from build123d import *

# Parameters (mm, degrees)
FILLET1_R          = 0.508
CHAMFER1_SIZE      = 0.508
CHAMFER1_SIZE2     = 0.87988181
SKETCH4_W          = 19.05
SKETCH4_H          = 3.175
CUT_EXTRUDE1_DEPTH = 4.7625
FILLET2_R          = 1.5875


with BuildPart() as part:
    # Sketch3 → Revolve1 (revolve)
    with BuildSketch(Plane(origin=(0, 0, 0), x_dir=(0, 0, -1), z_dir=(1, 0, 0)), mode=Mode.PRIVATE) as revolve1_sk:
        with BuildLine():
            Line((0, 0), (3.175, 0))
            Line((3.175, 0), (3.175, -8.255))
            ThreePointArc((3.175, -8.255), (3.691804849, -12.180522558), (5.207, -15.838527241))
            Line((5.207, -15.838527241), (10.16, -24.417374891))
            ThreePointArc((10.16, -24.417374891), (12.91700332, -28.010371571), (16.51, -30.767374891))
            Line((16.51, -30.767374891), (19.05, -32.233844575))
            Line((19.05, -32.233844575), (19.05, -34.265844575))
            Line((19.05, -34.265844575), (0, -34.265844575))
            Line((0, -34.265844575), (0, 0))
        make_face()
    revolve(revolve1_sk.sketch.rotate(Axis((0, 0, 0), (0, -1, 0)), 180), axis=Axis((0, 0, 0), (0, -1, 0)))

    # Fillet1
    fillet1_edges = [part.edges().sort_by_distance(p)[0] for p in [
        (0, -32.233844575, -19.05),
        (0, -34.265844575, -19.05),
    ]]
    fillet(fillet1_edges, radius=FILLET1_R)

    # Chamfer1
    chamfer1_edges = [part.edges().sort_by_distance(p)[0] for p in [
        (0, 0, -3.175),
    ]]
    chamfer1_side = [part.faces().sort_by_distance(p)[0] for p in [
        (0, -4.1275, -3.175),
    ]]
    chamfer(chamfer1_edges, length=CHAMFER1_SIZE, length2=CHAMFER1_SIZE2, reference=chamfer1_side[0])

    # Sketch4 → Cut-Extrude1 (cut)
    with BuildSketch(Plane.XZ.offset(34.265844575)):
        Rectangle(SKETCH4_W, SKETCH4_H)
    extrude(amount=-CUT_EXTRUDE1_DEPTH, mode=Mode.SUBTRACT)

    # Fillet2
    fillet2_edges = [part.edges().sort_by_distance(p)[0] for p in [
        (-9.525, -31.884594575, -1.5875),
        (9.525, -31.884594575, -1.5875),
        (9.525, -31.884594575, 1.5875),
        (-9.525, -31.884594575, 1.5875),
    ]]
    fillet(fillet2_edges, radius=FILLET2_R - 0.0001)  # a hair under: the kernel refuses the full size


solid = part.part
For this review, take the finished solid that the model builds, in its own axes (mm). A direction names the side the tool comes from. Give positions to 0.01 mm unless a question says otherwise; leave off trailing zeros. Loops run counter-clockwise (first coordinate to the right, second up) from the corner with the lowest first, then second, coordinate; pieces in that order, holes last.
Item 1: Draft analysis for pull direction X (two halves, no side actions). For faces 1 (the flat face through (0, -34.266, 4)), 2 (the flat face through (0, -32, 1.588)), 3 (the conical face through (3.36, -16.38, -4.38)), state which applies: +X half, -X half, draft (parallel to the pull), parting line (faces both ways), or undercut.
Item 2: Tool access review of faces 4 (the cylindrical face through (9.05, -31.85, -1.13)), 5 (the flat face through (0, 0, 0)), 6 (the cylindrical face through (2.8, -4.4, 1.5)): name each direction out of +Z, -Z, +X, -X, +Y, -Y from which nothing blocks a thin tool from reaching the whole face with its end or side.
Item 3: For line 1 along Z through (x, y) = (-8.5, -31.5); line 2 along X through (y, z) = (-27, -2); line 3 along Y through (x, z) = (-1, 16.5), list the stretches that pass through material, from the lowest coordinate up.
Item 4: Take a section at B-B, the plane y = -10. State the section outline as (x, z) points.
Item 5: Insertion check: pin 1 (5 mm diameter, centred on x = -1.5, y = -32.5, fed in from -Z); pin 2 (4 mm diameter, centred on x = -7, y = -10, fed in from +Z); pin 3 (10 mm diameter, centred on y = -30, z = -12.5, fed in from -X); pin 4 (1.5 mm diameter, centred on y = -17, z = -2.5, fed in from -X). Each pin has a flat end and moves straight along its axis. Give the tip position at first contact, or say it passes through.
Item 6: Take a section at A-A, the plane y = -6. State the section outline as (x, z) points (3 decimals), and give its area (3 significant figures).
Calculated:
1. face 1: draft
1. face 2: undercut
1. face 3: parting line
2. face 4: -Y
2. face 5: +Z, -Z, +X, -X, +Y
2. face 6: +Y
3. line 1: z = -15.62 to -1.48, 1.48 to 15.62
3. line 2: x = -11.82 to 11.82
3. line 3: y = -34.27 to -30.78
4. outline: circle Ø6.55 at (0, 0)
5. pin 1: stops at z = -19.05
5. pin 2: passes through
5. pin 3: stops at x = -17.22
5. pin 4: stops at x = -5.88
6. outline: circle Ø6.35 at (0, 0)
6. area: 31.7 mm2
